Source: CAD feature listing. Evaluate the final solid. Frame: model axes, mm. Face numbers are marked on the shaded views. A direction names the side the tool comes from. Round coordinates to 2 decimals unless told otherwise and drop trailing zeros. Loops run counter-clockwise (first coordinate to the right, second up) from the corner with the lowest first, then second, coordinate; pieces in that order, holes last. Notation, with made-up numbers: (-25, 29) -> (-15, 29) arc R18 cw to (-15, 41) -> close; hole circle Ø9 at (41.5, 47). An arc over 180 degrees is marked (long way). Put each result on its own line as item: value. Start each with the question number.
1. Material intervals for L1, parallel to Z at x = -35, y = 8; L2, parallel to Z at x = 19.5, y = 10; L3, parallel to Z at x = 14.5, y = -3, sorted ascending.
2. Cut plane B-B (y = -4.5). Return the cut outline in (x, z).
3. Cut plane A-A (x = -42.5). Return the cut outline in (y, z).
4. Draft query along Y for the marked faces 1, 2 and 3. Return one class per face: pulls with the +Y half, pulls with the -Y half, needs draft (parallel to the pull), parting line crosses it, or undercut.
5. Cut plane D-D (x = 0). Return the cut outline in (y, z), then the cut area to 4 significant figures.
6. Cut plane C-C (z = -3). Return the cut outline in (x, y), then the cut area to 3 significant figures.
7. Contact query for flat-ended pins moving along their axis: pin 1 (1 mm diameter, centred on x = 27, z = 7, fed in from -Y); pin 2 (5.5 mm diameter, centred on x = -28.5, y = 8, fed in from +Z); pin 3 (8 mm diameter, centred on x = 42, z = -3, fed in from +Y). Output: stop coordinate, or through.
8. Set-up query: the marked faces 4, 5, 6 and 7. Return all of +Z, -Z, +X, -X, +Y, -Y with unobstructed straight access to the full face (end or side cutting, diameter ignored); none if empty.
```python
from build123d import *

# Parameters (mm, degrees)
SKETCH1_W                = 12
SKETCH1_H                = 9
BOSS_EXTRUDE1_DEPTH      = 2.5
SKETCH2_W                = 17
SKETCH2_H                = 25
BOSS_EXTRUDE2_DEPTH      = 10
SKETCH4_W                = 15
SKETCH4_H                = 8
CUT_EXTRUDE1_DEPTH       = 42
SKETCH7_W                = 14
SKETCH7_H                = 12
BOSS_EXTRUDE3_DEPTH      = 72
SKETCH8_R                = 0.75
CUT_EXTRUDE2_DEPTH       = 72
SKETCH9_W                = 22
SKETCH9_H                = 12
CUT_EXTRUDE3_DEPTH       = 37
SKETCH5_R                = 2.5
CUT_EXTRUDE6_DEPTH       = 23.5
SKETCH12_W               = 47
SKETCH12_H               = 15
BOSS_EXTRUDE4_DEPTH      = 20
SKETCH13_W               = 45
SKETCH13_H               = 21.5
CUT_EXTRUDE7_DEPTH       = 14
SKETCH14_W               = 47
SKETCH14_H               = 4.916428424
BOSS_EXTRUDE5_DEPTH      = 20
SKETCH15_W               = 45
SKETCH15_H               = 3.916428424
CUT_EXTRUDE8_DEPTH       = 20
SKETCH16_W               = 30
SKETCH16_H               = 16
BOSS_EXTRUDE6_DEPTH      = 7
SKETCH17_W               = 14
SKETCH17_H               = 6
CUT_EXTRUDE9_DEPTH       = 100
CUT_EXTRUDE10_DEPTH      = 46.5
CUT_EXTRUDE10_DEPTH_BACK = 24.5
SKETCH19_W               = 12
SKETCH19_H               = 11
SKETCH21_R               = 4
CUT_EXTRUDE11_DEPTH      = 24.5


with BuildPart() as part:
    # Sketch1 → Boss-Extrude1 (new body)
    with BuildSketch(Plane(origin=(0, 0, 0), x_dir=(1, 0, 0), z_dir=(0, 1, 0))):
        Polygon((-50, -40.45305067), (-50, -50), (50, -50), (50, -40.45305067), (36, -40.45305067), (36, -16.45305067), (50, -16.45305067), (50, 50), (-50, 50), (-50, -16.45305067), (-36, -16.45305067), (-36, -40.45305067), align=None)
        with Locations((0, 40.5)):
            Rectangle(SKETCH1_W, SKETCH1_H, mode=Mode.SUBTRACT)
    extrude(amount=BOSS_EXTRUDE1_DEPTH)

    # Sketch2 → Boss-Extrude2 (add)
    with BuildSketch(Plane(origin=(0, 2.5, 0), x_dir=(1, 0, 0), z_dir=(0, 1, 0))):
        with Locations((-18.083526834, 37.5)):
            Rectangle(SKETCH2_W, SKETCH2_H)
    extrude(amount=BOSS_EXTRUDE2_DEPTH)

    # Sketch4 → Cut-Extrude1 (cut)
    with BuildSketch(Plane.XY.offset(-25)):
        with Locations((-18.083526834, 6.5)):
            Rectangle(SKETCH4_W, SKETCH4_H)
    extrude(amount=-CUT_EXTRUDE1_DEPTH, mode=Mode.SUBTRACT)

    # Sketch7 → Boss-Extrude3 (add)
    with BuildSketch(Plane.ZY.offset(36)):
        with Locations((28.45305067, 8.5)):
            Rectangle(SKETCH7_W, SKETCH7_H)
    extrude(amount=-BOSS_EXTRUDE3_DEPTH)

    # Sketch8 → Cut-Extrude2 (cut)
    with BuildSketch(Plane.ZY.offset(36)):
        with Locations((28.45305067, 8.5)):
            Circle(SKETCH8_R)
    extrude(amount=-CUT_EXTRUDE2_DEPTH, mode=Mode.SUBTRACT)

    # Sketch9 → Cut-Extrude3 (cut)
    with BuildSketch(Plane.XY.offset(35.45305067)):
        with Locations((0, 8.5)):
            Rectangle(SKETCH9_W, SKETCH9_H)
    extrude(amount=-CUT_EXTRUDE3_DEPTH, mode=Mode.SUBTRACT)

    # Sketch5 → Cut-Extrude6 (cut)
    with BuildSketch(Plane(origin=(0, 2.5, 0), x_dir=(1, 0, 0), z_dir=(0, 1, 0))):
        with Locations(Location((-18.083526834, 18.209316503, 0), (0, 0, 270))):
            Circle(SKETCH5_R)
    extrude(amount=-CUT_EXTRUDE6_DEPTH, mode=Mode.SUBTRACT)

    # Sketch12 → Boss-Extrude4 (add)
    with BuildSketch(Plane.XZ):
        with Locations((0, 42.5)):
            Rectangle(SKETCH12_W, SKETCH12_H)
    extrude(amount=BOSS_EXTRUDE4_DEPTH)

    # Sketch13 → Cut-Extrude7 (cut)
    with BuildSketch(Plane.XY.offset(50)):
        with Locations((0, -8.25)):
            Rectangle(SKETCH13_W, SKETCH13_H)
    extrude(amount=-CUT_EXTRUDE7_DEPTH, mode=Mode.SUBTRACT)

    # Sketch14 → Boss-Extrude5 (add)
    with BuildSketch(Plane.XZ):
        with Locations((0, -47.541785788)):
            Rectangle(SKETCH14_W, SKETCH14_H)
    extrude(amount=BOSS_EXTRUDE5_DEPTH)

    # Sketch15 → Cut-Extrude8 (cut)
    with BuildSketch(Plane.XZ.offset(20)):
        with Locations((0, -48.041785788)):
            Rectangle(SKETCH15_W, SKETCH15_H)
    extrude(amount=-CUT_EXTRUDE8_DEPTH, mode=Mode.SUBTRACT)

    # Sketch16 → Boss-Extrude6 (add)
    with BuildSketch(Plane(origin=(0, 2.5, 0), x_dir=(1, 0, 0), z_dir=(0, 1, 0))):
        with Locations((-35, 0)):
            Rectangle(SKETCH16_W, SKETCH16_H)
        with Locations((35, 0)):
            Rectangle(SKETCH16_W, SKETCH16_H)
    extrude(amount=BOSS_EXTRUDE6_DEPTH)

    # Sketch17 → Cut-Extrude9 (cut)
    with BuildSketch(Plane.ZY.offset(50)):
        with Locations((0, 5.5)):
            Rectangle(SKETCH17_W, SKETCH17_H)
    extrude(amount=-CUT_EXTRUDE9_DEPTH, mode=Mode.SUBTRACT)

    # Sketch19 → Cut-Extrude10 (cut, two sides: drawn at the far end of the back side and taken through both)
    with BuildSketch(Plane(origin=(-11, 0, 0), x_dir=(0, 0, -1), z_dir=(1, 0, 0)).offset(-CUT_EXTRUDE10_DEPTH_BACK)):
        with Locations((-28.45305067, 8)):
            Rectangle(SKETCH19_W, SKETCH19_H)
    extrude(amount=CUT_EXTRUDE10_DEPTH + CUT_EXTRUDE10_DEPTH_BACK, mode=Mode.SUBTRACT)

    # Sketch21 → Cut-Extrude11 (cut)
    with BuildSketch(Plane(origin=(0, 2.5, 0), x_dir=(1, 0, 0), z_dir=(0, 1, 0))):
        with Locations(Location((0, -29.805394333, 0), (0, 0, 270))):
            Circle(SKETCH21_R)
    extrude(amount=-CUT_EXTRUDE11_DEPTH, mode=Mode.SUBTRACT)


solid = part.part
```
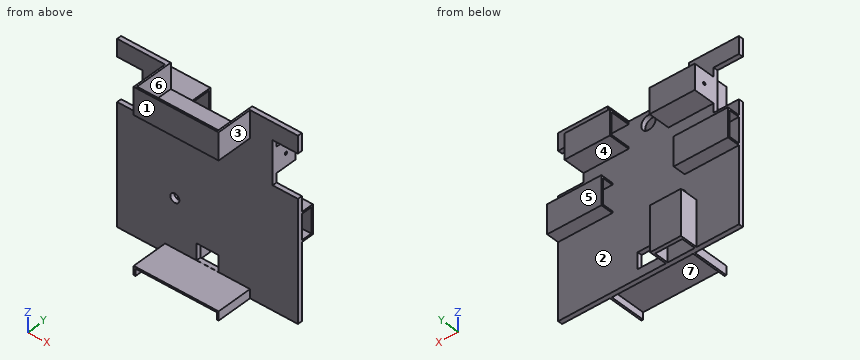
Solution:
1. L1: z = -8 to -7, 7 to 8, 21.45 to 22.45, 34.45 to 35.45
1. L2: z = 21.45 to 22.45, 34.45 to 35.45
1. L3: z = -46.08 to -45.08, 35 to 36
2. outline: (-23.5, -50) -> (-22.5, -50) -> (-22.5, -46.08) -> (22.5, -46.08) -> (22.5, -50) -> (23.5, -50) -> (23.5, -45.08) -> (-23.5, -45.08) -> close; (-23.5, 35) -> (23.5, 35) -> (23.5, 50) -> (22.5, 50) -> (22.5, 36) -> (-22.5, 36) -> (-22.5, 50) -> (-23.5, 50) -> close
3. outline: (0, -50) -> (2.5, -50) -> (2.5, -8) -> (9.5, -8) -> (9.5, 8) -> (2.5, 8) -> (2.5, 16.45) -> (0, 16.45) -> close; (0, 40.45) -> (2.5, 40.45) -> (2.5, 50) -> (0, 50) -> close; hole (2.5, -7) -> (8.5, -7) -> (8.5, 7) -> (2.5, 7) -> close
4. face 1: pulls with the -Y half
4. face 2: undercut
4. face 3: needs draft
5. outline: (-20, -46.08) -> (0, -46.08) -> (0, -50) -> (2.5, -50) -> (2.5, -45) -> (0, -45) -> (0, -45.08) -> (-20, -45.08) -> close; (-20, 35) -> (0, 35) -> (0, 33.81) -> (2.5, 33.81) -> (2.5, 36) -> (-19, 36) -> (-19, 50) -> (-20, 50) -> close; (0, -36) -> (2.5, -36) -> (2.5, 25.81) -> (0, 25.81) -> close
5. area: 226.5 mm^2
6. outline: (-50, 0) -> (50, 0) -> (50, 2.5) -> (-50, 2.5) -> close; (-50, 8.5) -> (-20, 8.5) -> (-20, 9.5) -> (-50, 9.5) -> close; (20, 8.5) -> (50, 8.5) -> (50, 9.5) -> (20, 9.5) -> close
6. area: 310 mm^2
7. pin 1: stops at y = 0
7. pin 2: stops at z = 35.45
7. pin 3: stops at y = 9.5
8. face 4: +X, -X, +Y
8. face 5: -Z, +X, -X, +Y
8. face 6: +Z, +Y
8. face 7: -Z, -Y
